Source: three-view drawing plus pictorial views. Frame: mm from the lowest corner of the part. A direction names the side the tool comes from. Round coordinates to 2 decimals unless told otherwise and drop trailing zeros. Order: outer loops, then holes, each group sorted by start corner. A loop starts at its lowest first (then second) coordinate and runs counter-clockwise, first axis right, second up. Notation, with made-up numbers: M 68.5,-34 L 114.5,-34 A15 cw 114.5,-5 Z; hole C -9,22 d7. An arc over 180 degrees is marked long. Return JSON: item names as keys, results as strings. Group by question number.
Q1. Contact query for flat-ended pins moving along their axis: pin 1 (3 mm diameter, centred on x = 22, y = 40.5, fed in from +Z); pin 2 (3.5 mm diameter, centred on x = 5, z = 2, fed in from -Y); pin 3 (1 mm diameter, centred on x = 13.5, z = 3, fed in from +Y). Output: stop coordinate, or through.
Q2. Mould query, pull axis Y, two halves, no side actions, for the marked faces 1, 2 and 3. Classes: released by +Y, released by -Y, zero draft, split by the parting line, or undercut.
Q3. Cut plane A-A on y = 31.5. Output: boundary loops of the cut face in (x, z).
Q4. Ray query, probe 1 along Y at (x, z) = (9.5, 3.25); probe 2 along Y at (x, z) = (32.5, 6.25); probe 3 along X at (y, z) = (18.5, 3) (1 decimal). Return the intervals inside material, ascending.
Q5. Cut plane C-C on z = 5. Count the separate pieces of the cut face and the enclosed holes in it, and give its area (3 significant figures).
Q6. Access query for the marked faces 4 and 5. Directions: +Z, -Z, +X, -X, +Y, -Y. A direction counts if a zero-diameter tool reaches every point of the face in a straight line with its end or side. Return the directions, or none.
Q7. Cut plane B-B on x = 9. Output: boundary loops of the cut face in (y, z).
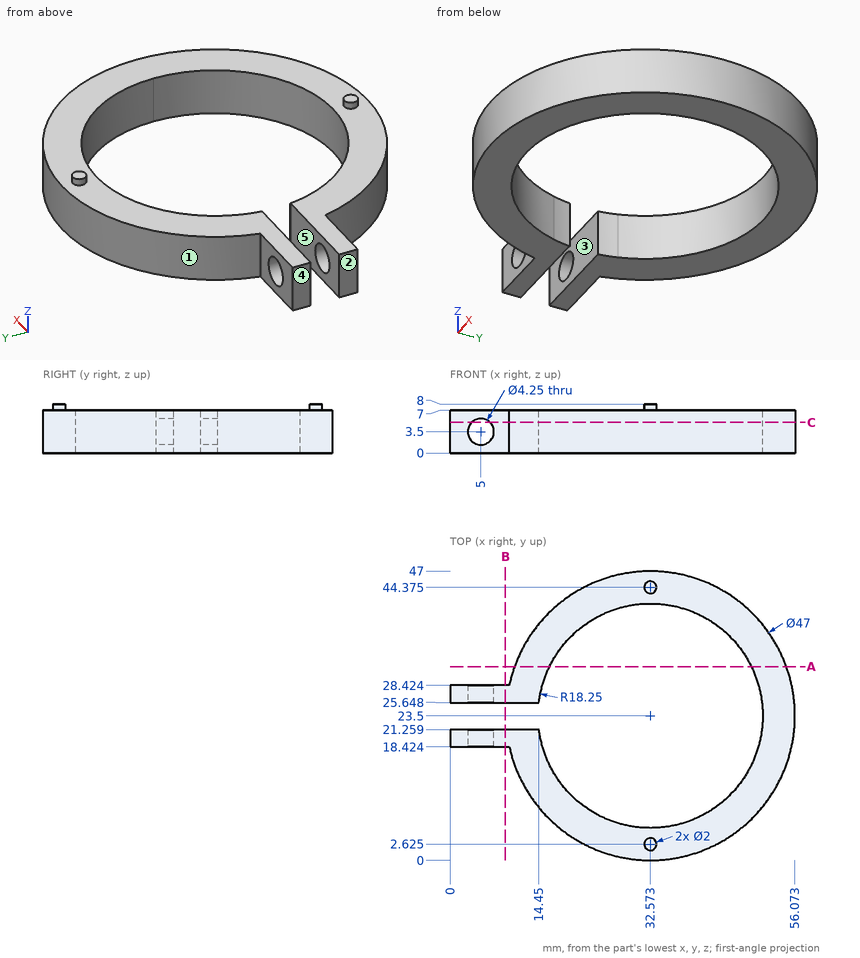
Result sheet:
{
 "1": {"pin 1": "stops at z = 7", "pin 2": "stops at y = 18.42", "pin 3": "stops at y = 37.9"},
 "2": {"face 1": "split by the parting line", "face 2": "zero draft", "face 3": "undercut"},
 "3": {"outline": "M 10.48,0 L 16.17,0 L 16.17,7 L 10.48,7 Z; M 48.98,0 L 54.67,0 L 54.67,7 L 48.98,7 Z"},
 "4": {"probe 1": "y = 18.42 to 21.26, 25.65 to 28.42", "probe 2": "y = 0 to 5.25, 41.75 to 47", "probe 3": "x = 0 to 2.9, 7.1 to 15, 50.1 to 55.5"},
 "5": {"separate pieces": "3", "enclosed holes": "0", "area": "701 mm²"},
 "6": {"face 4": "+Z, -Z, -X, +Y, -Y", "face 5": "+Z, -Z, -X"},
 "7": {"outline": "M 18.42,0 L 21.26,0 L 21.26,7 L 18.42,7 Z; M 25.65,0 L 28.42,0 L 28.42,7 L 25.65,7 Z"}
}
